For this review, take the finished solid that the model builds, in its own axes (mm). Coordinates: 2 decimals unless noted, no trailing zeros. Write each loop counter-clockwise with the first axis right and the second up, starting at its lowest first coordinate (ties: lowest second). Pieces come first, ordered by that corner, then holes. Notation, with made-up numbers: M -6.75,-26.75 L 43.25,-26.75 A23 ccw 43.25,-5.75 Z; hole C -20.75,19.5 d5. An arc over 180 degrees is marked long. One line per question, with ' | ' between items.
from build123d import *

# Parameters (mm, degrees)
EXTRUDE_1_DEPTH = 90
FILLET_1_R      = 5


with BuildPart() as part:
    # 草图1 → 凸台-拉伸1 (new body)
    with BuildSketch(Plane(origin=(0, 0, 0), x_dir=(1, 0, 0), z_dir=(0, 1, 0))):
        Polygon((0, 0), (16.378660542, -45), (26.378660542, -45), (26.378660542, 0), align=None)
    extrude(amount=EXTRUDE_1_DEPTH)

    # 圆角1
    fillet_1_edges = [part.edges().sort_by_distance(p)[0] for p in [
        (26.378660542, 45, 0),
    ]]
    fillet(fillet_1_edges, radius=FILLET_1_R)


solid = part.part
1. For line 1 along Z through (x, y) = (22, 14.5); line 2 along X through (y, z) = (12, 14); line 3 along X through (y, z) = (17.5, 28.5), list the stretches that pass through material, from the lowest coordinate up.
Computed values:
line 1: z = 0.04 to 45 | line 2: x = 5.1 to 26.38 | line 3: x = 10.37 to 26.38
2. Take a section at C-C on x = 3.75. State the section outline as (y, z) points.
Computed values:
outline: M 0,0 L 90,0 L 90,10.3 L 0,10.3 Z
3. Take a section at A-A on y = 68.5. State the section outline as (x, z) points, plus the area to 3 significant figures.
Computed values:
outline: M 0,0 L 21.38,0 A5 ccw 26.38,5 L 26.38,45 L 16.38,45 Z | area: 813 mm2
4. Clearance check with flat-ended pins moving along their axes: P1, Ø12, axis at y = 29, z = 19.5, coming from the -X side; P2, Ø2, axis at y = 21.5, z = 17, coming from the -X side; P3, Ø4, axis at x = 16, y = 43.5, coming from the +Z side; P4, Ø10, axis at y = 70, z = 24, coming from the -X side. State where each tip first meets the part, or that it passes through.
Computed values:
P1: stops at x = 4.91 | P2: stops at x = 5.82 | P3: stops at z = 45 | P4: stops at x = 6.92
5. Take a section at B-B on z = 24. State the section outline as (x, y) points.
Computed values:
outline: M 8.74,0 L 26.38,0 L 26.38,90 L 8.74,90 Z
